The listing builds one solid part. Answer for the finished solid, in the listing's coordinates (mm). A direction names the side the tool comes from. Round coordinates to 2 decimals unless told otherwise and drop trailing zeros. Order: outer loops, then holes, each group sorted by start corner. A loop starts at its lowest first (then second) coordinate and runs counter-clockwise, first axis right, second up. Notation, with made-up numbers: (21, -1.75) - (58, -1.75) arc R23 cw to (58, 35.25) - close; hole circle Ø3 at (35, 20.25). An arc over 180 degrees is marked (long way). One line per item, written item: value. Start each with the question number.
1. Section C-C, the plane z = 660 is taken. Give the vertices of the cut face in (x, y), then the cut area to 3 significant figures.
2. For a pull along X with two mould halves and no side action, classify faces 3 (the flat face through (-25, 0, 1232)), 4 (the flat face through (25, 0, 1232)), 5 (the flat face through (0, 21.8, 1268)) as released by +X, released by -X, zero draft, split by the parting line, or undercut.
3. Section A-A, the plane y = 10.5 is taken. Give the vertices of the cut face in (x, z).
4. Straight lines are drawn through the part: line 1 (X direction, y = -16, z = 1427); line 2 (X direction, y = -23, z = 1841). For each, find the intervals that lie inside material, in ascending order.
5. A tool of negligible diameter and unlimited length cuts with its end or side. For faces 1 (the flat face through (-21.8, 0, 1268)), 2 (the flat face through (0, 25, 1232)), from which of +Z, -Z, +X, -X, +Y, -Y can it reach the whole face along a straight path? Write none if from no direction.
from build123d import *

# Parameters (mm, degrees)
F0_W     = 50
F0_H     = 50
F1_DEPTH = 2500
F2_W     = 43.6
F2_H     = 43.6
F3_DEPTH = 2500.001
F4_R     = 3
F5_R     = 1


with BuildPart() as f1:
    # F0 (on Top) → F1 (new body)
    with BuildSketch(Plane.XY):
        Rectangle(F0_W, F0_H)
    extrude(amount=F1_DEPTH)

    # F2 (on face) → F3 (cut, through all)
    with BuildSketch(Plane.XY.offset(2500)):
        Rectangle(F2_W, F2_H)
    extrude(amount=-F3_DEPTH, mode=Mode.SUBTRACT)

    # F4
    f4_edges = [f1.edges().sort_by_distance(p)[0] for p in [
        (25, -25, 1250),
        (25, 25, 1250),
        (-25, -25, 1250),
        (-25, 25, 1250),
    ]]
    fillet(f4_edges, radius=F4_R)

    # F5
    f5_edges = [f1.edges().sort_by_distance(p)[0] for p in [
        (21.8, -21.8, 1250),
        (-21.8, 21.8, 1250),
        (21.8, 21.8, 1250),
        (-21.8, -21.8, 1250),
    ]]
    fillet(f5_edges, radius=F5_R)


solid = f1.part
Answer list:
1. outline: (-25, -22) arc R3 ccw to (-22, -25) - (22, -25) arc R3 ccw to (25, -22) - (25, 22) arc R3 ccw to (22, 25) - (-22, 25) arc R3 ccw to (-25, 22) - close; hole (-21.8, -20.8) arc R1 ccw to (-20.8, -21.8) - (20.8, -21.8) arc R1 ccw to (21.8, -20.8) - (21.8, 20.8) arc R1 ccw to (20.8, 21.8) - (-20.8, 21.8) arc R1 ccw to (-21.8, 20.8) - close
1. area: 592 mm²
2. face 3: released by -X
2. face 4: released by +X
2. face 5: undercut
3. outline: (-25, 0) - (-21.8, 0) - (-21.8, 2500) - (-25, 2500) - close; (21.8, 0) - (25, 0) - (25, 2500) - (21.8, 2500) - close
4. line 1: x = -25 to -21.8, 21.8 to 25
4. line 2: x = -24.83 to 24.83
5. face 1: +Z, -Z
5. face 2: +Z, -Z, +X, -X, +Y
